Answer from the drawing. Dimensions are ordinates in mm from the lowest x, y and z of the part. A direction names the side the tool comes from. Round coordinates to 2 decimals unless told otherwise and drop trailing zeros. Write each loop counter-clockwise with the first axis right and the second up, starting at its lowest first coordinate (ties: lowest second). Pieces come first, ordered by that corner, then holes. Notation, with made-up numbers: (1.5, 18) - (41.5, 18) arc R17 ccw to (41.5, 45) - close; hole circle Ø6 at (-7, 17). An arc over 180 degrees is marked (long way). Write item = value, one per line. Start each with the question number.
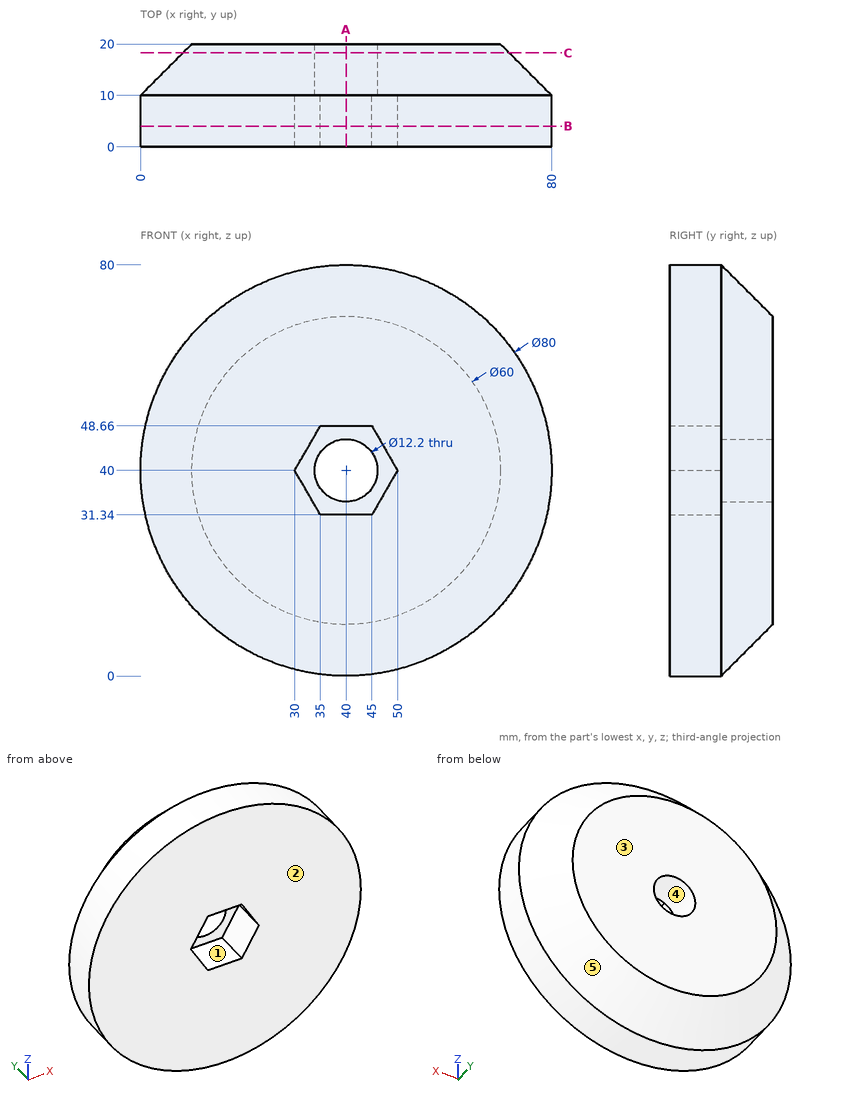
1. Consider line 1 (X direction, y = 12, z = 40); line 2 (Z direction, x = 40, y = 13); line 3 (X direction, y = 12.25, z = 40). Determine where each line is inside the solid, lowest interval first.
2. Find section B-B on y = 4. Give the vertices of the cut face in (x, z).
3. For a pull along X with two mould halves and no side action, classify the marked faces 3, 4 and 5 as released by +X, released by -X, zero draft, split by the parting line, or undercut.
4. Find section A-A on x = 40. Give the vertices of the cut face in (y, z).
5. Which of the six approach directions +Z, -Z, +X, -X, +Y, -Y give full straight-line access (tool end or side, diameter ignored) to the marked faces 1 and 2?
6. Find section C-C on y = 18.25. Give the vertices of the cut face in (x, z), plus the area to 3 significant figures.
7. Each of these flat-tipped pins is pushed along its axis until it touches: pin 1 (16 mm diameter, centred on x = 40, z = 40, fed in from -Y); pin 2 (3 mm diameter, centred on y = 16, z = 28.5, fed in from -X) (1 decimal); pin 3 (11 mm diameter, centred on x = 41.5, y = 6, fed in from +Z). Where does it stop, or does it pass through?
Answer key:
q1.line_1 = 2 to 33.9, 46.1 to 78
q1.line_2 = 3 to 33.9, 46.1 to 77
q1.line_3 = 2.25 to 33.9, 46.1 to 77.75
q2.outline = circle Ø80 at (40, 40); hole (30, 40) - (35, 31.34) - (45, 31.34) - (50, 40) - (45, 48.66) - (35, 48.66) - close
q3.face_3 = zero draft
q3.face_4 = undercut
q3.face_5 = split by the parting line
q4.outline = (0, 0) - (10, 0) - (20, 10) - (20, 33.9) - (10, 33.9) - (10, 31.34) - (0, 31.34) - close; (0, 48.66) - (10, 48.66) - (10, 46.1) - (20, 46.1) - (20, 70) - (10, 80) - (0, 80) - close
q5.face_1 = -Y
q5.face_2 = +Z, -Z, +X, -X, -Y
q6.outline = circle Ø63.5 at (40, 40); hole circle Ø12.2 at (40, 40)
q6.area = 3,050 mm²
q7.pin_1 = 10
q7.pin_2 = 6.3
q7.pin_3 = 80
